Source: CAD feature listing. Evaluate the final solid. Frame: model axes, mm. A direction names the side the tool comes from. Give positions to 0.01 mm unless a question says otherwise; leave off trailing zeros. Loops run counter-clockwise (first coordinate to the right, second up) from the corner with the lowest first, then second, coordinate; pieces in that order, holes last.
from build123d import *

# Parameters (mm, degrees)
F1_W     = 76.2
F1_H     = 76.2
F1_W_2   = 63.5
F1_H_2   = 63.5
F2_DEPTH = 451.32752
F3_R     = 7.14375
F4_DEPTH = 76.201


# Not quite as in the source:
# - a variable given as a bare number and used for a length is read in inches; the dataset says mm whatever the document's units were


with BuildPart() as f2:
    # F1 (on Right) → F2 (new body)
    with BuildSketch(Plane.YZ):
        Rectangle(F1_W, F1_H)
        Rectangle(F1_W_2, F1_H_2, mode=Mode.SUBTRACT)
    extrude(amount=F2_DEPTH)

    # F3 (on face) → F4 (cut, through all)
    with BuildSketch(Plane.XZ.offset(38.1)):
        with Locations((152.4, 0)):
            Circle(F3_R)
        with Locations((127.6604, 0)):
            Circle(F3_R)
    extrude(amount=-F4_DEPTH, mode=Mode.SUBTRACT)


solid = f2.part
1) Pull-direction query (Z, two-part tool) for faces 3 (the flat face through (223, -1, 38.1)), 4 (the cylindrical face through (159.214, -34.969, 2.146)), 5 (the flat face through (223, -38.1, -1)), 6 (the flat face through (223, -1, -38.1)); classes: released by +Z, released by -Z, zero draft, split by the parting line, or undercut.
Checks:
face 3: released by +Z
face 4: undercut
face 5: zero draft
face 6: released by -Z
2) Reachability of faces 1 (the flat face through (223, 31.75, 0)), 2 (the flat face through (451.328, -34, 1)) from +Z, -Z, +X, -X, +Y, -Y: full face, straight path, thin tool, end or side. Return the list, or none.
Checks:
face 1: +X, -X
face 2: +Z, -Z, +X, +Y, -Y
3) Ray query, probe 1 along Y at (x, z) = (267.5, 17); probe 2 along Z at (x, y) = (152.4, 36.75). Return the intervals inside material, ascending.
Checks:
probe 1: y = -38.1 to -31.75, 31.75 to 38.1
probe 2: z = -38.1 to -7.14, 7.14 to 38.1
4) Cut plane A-A (z = 24.5). Return loops of the section in (x, y), and give its area (3 significant figures).
Checks:
outline: (0, -38.1) - (451.33, -38.1) - (451.33, -31.75) - (0, -31.75) - close; (0, 31.75) - (451.33, 31.75) - (451.33, 38.1) - (0, 38.1) - close
area: 5,730 mm2
5) Contact query for a flat-ended pin moving along its axis: P1, Ø18.5, axis at x = 127.66, z = 0, coming from the +Y side. Output: stop coordinate, or through.
Checks:
P1: stops at y = 38.1
6) Cut plane C-C (z = 0). Return loops of the section in (x, y), and give its area (3 significant figures).
Checks:
outline: (0, -38.1) - (120.52, -38.1) - (120.52, -31.75) - (0, -31.75) - close; (0, 31.75) - (120.52, 31.75) - (120.52, 38.1) - (0, 38.1) - close; (134.8, -38.1) - (145.26, -38.1) - (145.26, -31.75) - (134.8, -31.75) - close; (134.8, 31.75) - (145.26, 31.75) - (145.26, 38.1) - (134.8, 38.1) - close; (159.54, -38.1) - (451.33, -38.1) - (451.33, -31.75) - (159.54, -31.75) - close; (159.54, 31.75) - (451.33, 31.75) - (451.33, 38.1) - (159.54, 38.1) - close
area: 5,370 mm2
7) Cut plane B-B (x = 152.4). Return loops of the section in (y, z), and give its area (3 significant figures).
Checks:
outline: (-38.1, -38.1) - (38.1, -38.1) - (38.1, -7.14) - (31.75, -7.14) - (31.75, -31.75) - (-31.75, -31.75) - (-31.75, -7.14) - (-38.1, -7.14) - close; (-38.1, 7.14) - (-31.75, 7.14) - (-31.75, 31.75) - (31.75, 31.75) - (31.75, 7.14) - (38.1, 7.14) - (38.1, 38.1) - (-38.1, 38.1) - close
area: 1,590 mm2
